Autodesk Inventor part; units mm, degrees
ref_plane "YZ Plane" through (0, 0, 0) normal (1, 0, 0) x (0, 1, 0)
ref_plane "XZ Plane" through (0, 0, 0) normal (0, 1, 0) x (-1, 0, 0)
ref_plane "XY Plane" through (0, 0, 0) normal (0, 0, 1) x (1, 0, 0)
sketch "スケッチ1" plane through (0, 0, 0) normal (0, 1, 0) x (-1, 0, 0)
  line L0 (-87.5, 105) -> (87.5, 105)
  line L1 (87.5, 105) -> (87.5, -105)
  line L2 (87.5, -105) -> (-87.5, -105)
  line L3 (-87.5, -105) -> (-87.5, 105)
  line L4 (-87.5, 105) -> (87.5, -105) construction
  line L5 (87.5, 105) -> (-87.5, -105) construction
  point P0 (0, 0)
  dimension "d0" = 210
  dimension "d1" = 175
extrude "プレート1" add sketch "スケッチ1" along normal blind 2
sketch "スケッチ5" plane through (0, 2, 0) normal (0, 1, 0) x (1, 0, 0)
  line L0 (-24, -101) -> (34.6, -101)
  line L1 (34.6, -101) -> (34.6, -67)
  line L2 (34.6, -67) -> (-24, -67)
  line L3 (-24, -67) -> (-24, -101)
  line L4 (-24, -101) -> (34.6, -67) construction
  line L5 (34.6, -101) -> (-24, -67) construction
  line L6 (87.5, -105) -> (-87.5, -105)
  point P0 (0, 0)
  point P1 (0, -84)
  point P2 (5.3, -84)
  point P3 (5.3, -84)
  dimension "d31" = 58.6
  dimension "d32" = 24
  dimension "d33" = 34
  dimension "d78" = 4
hole "穴3" at (34.6, 2, 67) at (34.6, 2, 101) at (-24, 2, 67) at (-24, 2, 101) direction (0, -1, 0) diameter 4.3 end through all
sketch "スケッチ6" plane through (0, 2, 0) normal (0, 1, 0) x (1, 0, 0)
  line L0 (-133.9967, -217.2896) -> (133.2896, 49.9967)
  line L1 (133.2896, 49.9967) -> (133.9967, 49.2896)
  line L2 (133.9967, 49.2896) -> (-133.2896, -217.9967)
  line L3 (-133.2896, -217.9967) -> (-133.9967, -217.2896)
  line L4 (-133.9967, -217.2896) -> (133.9967, 49.2896) construction
  line L5 (133.2896, 49.9967) -> (-133.2896, -217.9967) construction
  line L6 (133.9967, -217.2896) -> (-133.2896, 49.9967)
  line L7 (-133.2896, 49.9967) -> (-133.9967, 49.2896)
  line L8 (-133.9967, 49.2896) -> (133.2896, -217.9967)
  line L9 (133.2896, -217.9967) -> (133.9967, -217.2896)
  line L10 (133.9967, -217.2896) -> (-133.9967, 49.2896) construction
  line L11 (-133.2896, 49.9967) -> (133.2896, -217.9967) construction
  line L12 (-2.4749, -82.2322) -> (-1.7678, -81.5251)
  circle A0 centre (0, -84) radius 22
  line L13 (2.4749, -82.2322) -> (1.7678, -81.5251)
  circle A1 centre (0, -84) radius 3
  line L14 (-87.5, -105) -> (-87.5, 105)
  line L15 (87.5, 105) -> (87.5, -105)
  line L16 (122.5, 0) -> (-122.5, 0)
  point P0 (0, 0)
  point P1 (0, -84)
  point P2 (-2.1213, -81.8787)
  point P3 (2.1213, -81.8787)
  point P4 (15.9059, -68.8012)
  point P5 (-15.9059, -68.8012)
  dimension "d54" = 1
  dimension "d55" = 1
  dimension "d57" = 44
  dimension "d59" = 3
  dimension "d60" = 3
  dimension "d65" = 186
  dimension "d66" = 186
  dimension "d79" = 45
  dimension "d80" = 45
extrude "押し出し2" cut sketch "スケッチ6" against normal blind 10 contours A0 L6 L12 L8 | A0 L0 A1 L6 | L12 L6 A1 | A0 L2 L13 L0 | L0 L13 A1
sketch "スケッチ7" plane through (0, 2, 0) normal (0, 1, 0) x (1, 0, 0)
  line L0 (-82.5, -100) -> (82.5, -100)
  line L1 (82.5, -100) -> (82.5, 100)
  line L2 (82.5, 100) -> (-82.5, 100)
  line L3 (-82.5, 100) -> (-82.5, -100)
  line L4 (-82.5, -100) -> (82.5, 100) construction
  line L5 (82.5, -100) -> (-82.5, 100) construction
  line L6 (-87.5, -105) -> (-87.5, 105)
  line L7 (87.5, -105) -> (-87.5, -105)
  point P0 (0, 0)
  point P1 (-82.5, -45)
  point P2 (-82.5, -10)
  point P3 (82.5, -45)
  point P4 (82.5, -10)
  dimension "d45" = 5
  dimension "d46" = 5
  dimension "d67" = 55
  dimension "d68" = 35
  dimension "d69" = 55
  dimension "d70" = 35
hole "穴4" at (-82.5, 2, -100) at (82.5, 2, -100) at (-82.5, 2, 100) at (82.5, 2, 100) direction (0, -1, 0) diameter 3.2 end through all
sketch "スケッチ8" plane through (0, 2, 0) normal (0, 1, 0) x (1, 0, 0)
  line L0 (15.9059, -68.8012) -> (2.4749, -82.2322)
  line L1 (-2.1213, -81.8787) -> (-2.4749, -82.2322)
  arc A0 (2.1213, -81.8787) -> (-2.1213, -81.8787) centre (0, -84) ccw
  line L2 (2.4749, -82.2322) -> (2.1213, -81.8787)
  line L3 (-2.4749, -82.2322) -> (-15.9059, -68.8012)
  arc A1 (15.9059, -68.8012) -> (-15.9059, -68.8012) centre (0, -84) ccw
  line L4 (2.4749, -83.6464) -> (17.2895, -68.8318)
  arc A2 (17.2895, -68.8318) -> (-17.2895, -68.8318) centre (0, -84) ccw
  line L5 (-17.2895, -68.8318) -> (-2.4749, -83.6464)
  line L6 (-2.4749, -83.6464) -> (-1.4142, -82.5858)
  arc A3 (1.4142, -82.5858) -> (-1.4142, -82.5858) centre (0, -84) ccw
  line L7 (1.4142, -82.5858) -> (2.4749, -83.6464)
  point P0 (0, 0)
  dimension "d61" = 1
extrude "押し出し3" cut sketch "スケッチ8" against normal blind 10 contours L0 L2 A0 L1 L3 A1 | L7 A3 L6 L5 A2 L4
fillet "コーナーR1" radius 1 4 edges at (-2.4749, 1, 83.6464) (2.4749, 1, 83.6464) (-17.2895, 1, 68.8318) (17.2895, 1, 68.8318)
hole "穴5" at (-82.5, 2, 45) at (-82.5, 2, 10) at (82.5, 2, 45) at (82.5, 2, 10) direction (0, -1, 0) diameter 3.4 end through all
ref_plane "作業平面1" through (-87.5, 0, 20) normal (0, 0, 1) x (1, 0, 0)
sketch "スケッチ9" plane through (-87.5, 0, 20) normal (0, 0, 1) x (1, 0, 0)
  line L0 (175, 0) -> (175, 2)
  line L1 (0, 0) -> (175, 0)
  line L2 (175, 0) -> (175, 2)
  line L3 (175, 2) -> (0, 2)
  line L4 (0, 2) -> (0, 0)
  point P0 (87.5, 0)
extrude "押し出し4" cut sketch "スケッチ9" against normal blind 159
equation "\"d40\" = Thickness"
equation "\"d60\" = d59"
equation "\"d66\" = d65"
equation "\"d76\" = Thickness"
equation "\"d2\" = Thickness"
equation "\"BendRadius\" = Thickness"
equation "\"BendReliefWidth\" = Thickness"
equation "\"BendReliefDepth\" = 0.5 * Thickness"
equation "\"CornerReliefSize\" = 4 * Thickness"
equation "\"MinimumRemnant\" = 2 * Thickness"
equation "\"TransitionRadius\" = BendRadius"
equation "\"JacobiRadiusSize\" = BendRadius"
equation "\"GapSize\" = Thickness"
properties part number "s_carbon_plate1" material "CFRP"
Source: CAD feature listing. Evaluate the final solid. Frame: model axes, mm. A direction names the side the tool comes from. Round coordinates to 2 decimals unless told otherwise and drop trailing zeros. Loops run counter-clockwise (first coordinate to the right, second up) from the corner with the lowest first, then second, coordinate; pieces in that order, holes last. Notation, with made-up numbers: M 7.25,1.5 L 24.25,1.5 A10 ccw 24.25,6.5 Z; hole C 58.5,8 d11. An arc over 180 degrees is marked long. Return JSON: item names as keys, results as strings. Group by question number.
1. Section query A-A on z = 45. Output: boundary loops of the cut face in (x, y), and give its area (3 significant figures).
2. Material intervals for line 1 along X through (y, z) = (0.3, 45); line 2 along X through (y, z) = (0.95, 67); line 3 along X through (y, z) = (0.6, 101), sorted ascending. Write a range as from..to.
3. Reachability of faces 1 (the face through (1, 0, 54)), 2 (the face through (9.8, 1.01, 76.32)) from +Z, -Z, +X, -X, +Y, -Y: full face, straight path, thin tool, end or side. Return the list, or none.
4. Section query D-D on x = -5.5. Output: boundary loops of the cut face in (y, z).
5. Mould query, pull axis Z, two halves, no side actions, for faces 3 (the face through (1, 2, 54)), 4 (the face through (-81.47, 0.99, 43.65)). Classes: released by +Z, released by -Z, zero draft, split by the parting line, or undercut.
6. Section query B-B on x = -24. Output: boundary loops of the cut face in (y, z).
7. Section query C-C on y = 1.2. State how many separate pieces and enclosed holes the cut face has, and give its area (3 significant figures).
Checks:
{
 "1": {"outline": "M -87.5,0 L -84.2,0 L -84.2,2 L -87.5,2 Z; M -80.8,0 L 80.8,0 L 80.8,2 L -80.8,2 Z; M 84.2,0 L 87.5,0 L 87.5,2 L 84.2,2 Z", "area": "336 mm²"},
 "2": {"line 1": "x = -87.5..-84.2, -80.8..80.8, 84.2..87.5", "line 2": "x = -87.5..-26.15, -21.85..-15.49, 15.49..32.45, 36.75..87.5", "line 3": "x = -87.5..-83.75, -81.25..-26.15, -21.85..32.45, 36.75..81.25, 83.75..87.5"},
 "3": {"face 1": "+Z, -Z, +X, -X, -Y", "face 2": "+Y, -Y"},
 "4": {"outline": "M 0,20 L 2,20 L 2,61.67 L 0,61.67 Z; M 0,80.62 L 2,80.62 L 2,105 L 0,105 Z"},
 "5": {"face 3": "zero draft", "face 4": "undercut"},
 "6": {"outline": "M 0,20 L 2,20 L 2,64.85 L 0,64.85 Z; M 0,69.15 L 2,69.15 L 2,98.85 L 0,98.85 Z; M 0,103.15 L 2,103.15 L 2,105 L 0,105 Z"},
 "7": {"separate pieces": "1", "enclosed holes": "9", "area": "14,300 mm²"}
}
